Job drawing, mm, ordinate dimensions from the low corner. One solid piece. A direction names the side the tool comes from. Give positions to 0.01 mm unless a question says otherwise; leave off trailing zeros. Order: outer loops, then holes, each group sorted by start corner. A loop starts at its lowest first (then second) coordinate and runs counter-clockwise, first axis right, second up. Notation, with made-up numbers: (55.5, 11.5) - (75.5, 11.5) arc R25 cw to (75.5, 50.5) - close; hole circle Ø5 at (69.25, 80). An arc over 180 degrees is marked (long way). Write each question's results on one line, items separated by ' | '. Start each with the question number.
1) Cut at C-C on z = 161. List the corners of the cut face in (x, y), plus the area to 3 significant figures.
2) Cut at B-B on x = 298.5. List the corners of the cut face in (y, z), plus the area to 3 significant figures.
3) Drop flat-ended pins along their axis: pin 1 Ø12 at (x, z) = (393.5, 90.5) entering from -Y; pin 2 Ø1.5 at (x, y) = (358, 141.5) entering from -Z; pin 3 Ø5 at (y, z) = (92.5, 46) entering from +X. Give the stop position or say it passes through.
4) Two-plate mould, pull along Z, no slides. Class the marked faces 4, 5, 6 and 7: +Z half, -Z half, draft (parallel to the pull), parting line (faces both ways), or undercut.
5) Drill centre lines: line 1 along Z through (x, y) = (150.5, 81.5); line 2 along Y through (x, z) = (40, 46). Where is each one in solid material? Low to high. Write a range as from..to.
6) Tool access for the marked faces 1, 2 and 3: list every direction of +Z, -Z, +X, -X, +Y, -Y with a clear straight run to the whole face (end or side of a thin tool).
7) Cut at A-A on y = 68.5. List the corners of the cut face in (x, z), plus the area to 3 significant figures.
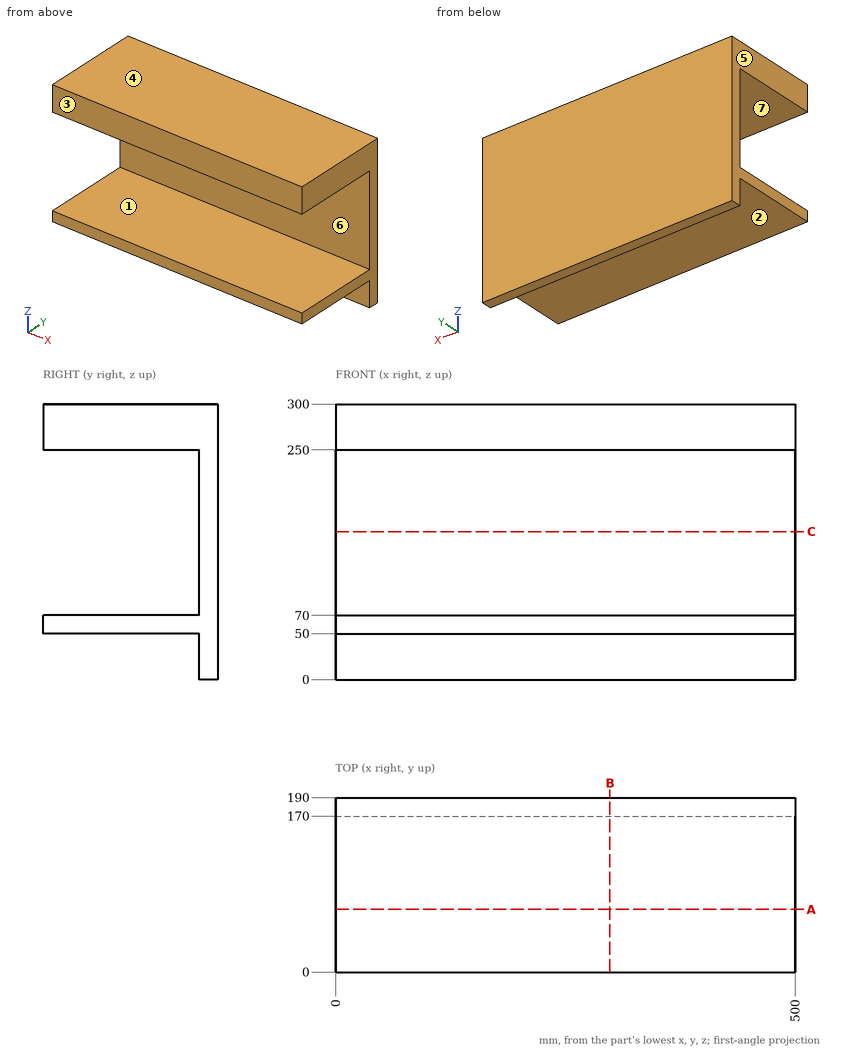
Results:
1) outline: (0, 170) - (500, 170) - (500, 190) - (0, 190) - close | area: 10,000 mm^2
2) outline: (0, 50) - (170, 50) - (170, 0) - (190, 0) - (190, 300) - (0, 300) - (0, 250) - (170, 250) - (170, 70) - (0, 70) - close | area: 17,900 mm^2
3) pin 1: y = 170 | pin 2: z = 50 | pin 3: through
4) face 4: +Z half | face 5: draft | face 6: undercut | face 7: undercut
5) line 1: 50..70, 250..300 | line 2: 170..190
6) face 1: +X, -X, -Y | face 2: -Z, +X, -X, -Y | face 3: +Z, -Z, +X, -X, -Y
7) outline: (0, 50) - (500, 50) - (500, 70) - (0, 70) - close; (0, 250) - (500, 250) - (500, 300) - (0, 300) - close | area: 35,000 mm^2
